For this review, take the finished solid that the model builds, in its own axes (mm). Give positions to 0.01 mm unless a question says otherwise; leave off trailing zeros. Write each loop counter-clockwise with the first axis right and the second up, starting at its lowest first coordinate (ties: lowest second). Pieces come first, ordered by that corner, then holes. Notation, with made-up numbers: M 75,83 L 104,83 A16 cw 104,88 Z; hole C 37,9.5 d6. An arc over 180 degrees is marked long. Use one line per item in the form item = value. Start each with the question number.
Q1. Consider section A-A on x = 683.75. Write out the cut boundary in (y, z).
Q2. Consider section B-B on y = 308.25. Write out the cut boundary in (x, z), and give its area (3 significant figures).
Q3. Consider section C-C on z = 0.9. Write out the cut boundary in (x, y).
Q4. For probe 1 along X at (y, z) = (287.75, 0.1); probe 2 along Y at (x, z) = (684.5, 0.85); probe 3 along Y at (x, z) = (704.5, 0.2), list the stretches that pass through material, from the lowest coordinate up. Write a range as [from, to].
Q5. Mouldability with a two-part tool opening along X and no side actions: class faces 1 (the cylindrical face through (702.37, 288.5, 0.59)), 2 (the flat face through (692.74, 297.67, 0.59)), 3 (the flat face through (694, 298, 0)) as released by +X, released by -X, zero draft, split by the parting line, or undercut.
Q6. Consider section D-D on y = 290.75. Write out the cut boundary in (x, z), and give its area (3 significant figures).
Q7. Clearance check with flat-ended pins moving along their axes: pin 1 Ø3 at (x, y) = (703.36, 287.74) entering from -Z; pin 2 Ø2 at (x, y) = (684.36, 308.74) entering from +Z. State where each tip first meets the part, or that it passes through.
Autodesk Inventor part; units mm, degrees
ref_plane "YZ Plane" through (0, 0, 0) normal (1, 0, 0) x (0, 1, 0)
ref_plane "XZ Plane" through (0, 0, 0) normal (0, 1, 0) x (-1, 0, 0)
ref_plane "XY Plane" through (0, 0, 0) normal (0, 0, 1) x (1, 0, 0)
sketch "Boceto1" plane through (0, 0, 0) normal (0, 0, 1) x (1, 0, 0)
  circle A0 centre (684.3626, 308.7393) radius 1.25
  arc A1 (686.7332, 307.9454) -> (684.4469, 306.2407) centre (684.3626, 308.7393) ccw
  circle A2 centre (703.3626, 287.7393) radius 1.25
  arc A3 (700.9878, 288.5205) -> (703.2626, 290.2373) centre (703.3626, 287.7393) ccw
  line L0 (684.3626, 308.7393) -> (703.3626, 287.7393) construction
  line L1 (689.4053, 303.1658) -> (691.9544, 305.4721) construction
  line L2 (686.8431, 307.4441) -> (702.8784, 290.3944)
  line L3 (684.828, 306.0836) -> (700.877, 289.0192)
  arc A4 (702.8784, 290.3944) -> (703.2626, 290.2373) centre (703.2426, 290.7369) ccw
  arc A5 (700.9878, 288.5205) -> (700.877, 289.0192) centre (700.5128, 288.6767) ccw
  arc A6 (686.7332, 307.9454) -> (686.8431, 307.4441) centre (687.2073, 307.7866) ccw
  arc A7 (684.828, 306.0836) -> (684.4469, 306.2407) centre (684.4637, 305.741) ccw
  point P0 (0, 0)
  point P1 (685.216, 309.1769)
  point P2 (703.1674, 288.8662)
  point P3 (683.8421, 307.9339)
  point P4 (702.2609, 288.0459)
  point P5 (686.6251, 307.6758)
  point P6 (684.6643, 306.2576)
  point P7 (701.0936, 288.7889)
  point P8 (703.0435, 290.2189)
  dimension "d7" = 2.5
  dimension "d8" = 5
  dimension "d10" = 5
  dimension "d11" = 19
  dimension "d12" = 21
  dimension "d14" = 2.4
  dimension "d15" = 0.5
extrude "Extrusión1" add sketch "Boceto1" along normal blind 1.2
properties part number "Pieza8_3DPrint"
Working result:
q1.outline = M 306.32,0 L 307.65,0 L 307.65,1.2 L 306.32,1.2 Z; M 309.83,0 L 311.16,0 L 311.16,1.2 L 309.83,1.2 Z
q2.outline = M 681.91,0 L 683.21,0 L 683.21,1.2 L 681.91,1.2 Z; M 685.51,0 L 686.81,0 L 686.81,1.2 L 685.51,1.2 Z
q2.area = 3.12 mm²
q3.outline = M 684.45,306.24 A0.5 cw 684.83,306.08 L 700.88,289.02 A0.5 cw 700.99,288.52 A2.5 ccw long 703.26,290.24 A0.5 cw 702.88,290.39 L 686.84,307.44 A0.5 cw 686.73,307.95 A2.5 ccw long Z; hole C 684.36,308.74 d2.5; hole C 703.36,287.74 d2.5
q4.probe_1 = [700.86, 702.11], [704.61, 705.86]
q4.probe_2 = [306.24, 307.5], [309.98, 311.24]
q4.probe_3 = [285.51, 287.22], [288.26, 289.97]
q5.face_1 = undercut
q5.face_2 = released by -X
q5.face_3 = zero draft
q6.outline = M 699.25,0 L 702.54,0 L 702.54,1.2 L 699.25,1.2 Z
q6.area = 3.95 mm²
q7.pin_1 = 0
q7.pin_2 = through
